The drawing under review shows one solid part. Ordinate dimensions are in mm from its lowest x, y, z. A direction names the side the tool comes from. Give positions to 0.01 mm unless a question says otherwise; leave off trailing zeros. Loops run counter-clockwise (first coordinate to the right, second up) from the corner with the lowest first, then second, coordinate; pieces in that order, holes last. Notation, with made-up numbers: M -38.5,44 L -16.5,44 A21 cw -16.5,78 Z; hole C -1,-9 d11. An arc over 180 degrees is marked long. Put each result on its own line as item: value. Start each with the question number.
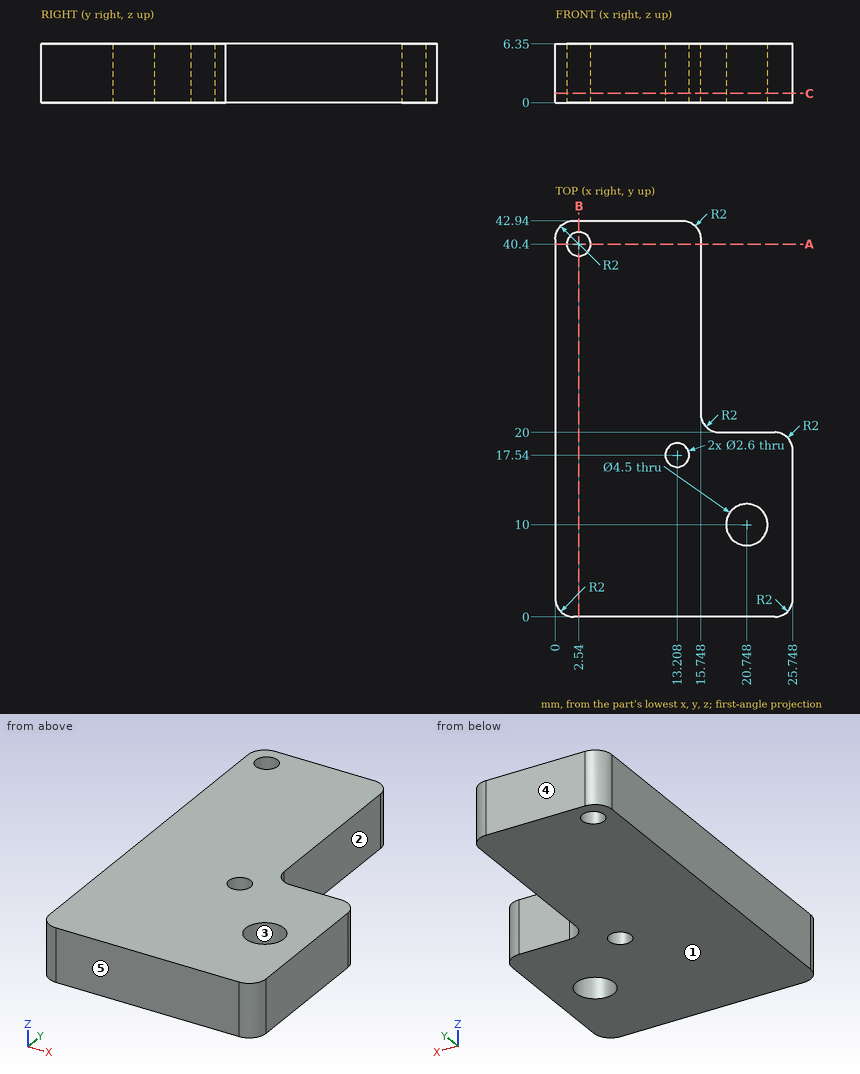
(1) Draft analysis for pull direction Y (two halves, no side actions). For the marked faces 3, 4 and 5, state which applies: +Y half, -Y half, draft (parallel to the pull), parting line (faces both ways), or undercut.
(2) To check wall thickness, follow L1, parallel to Y at x = 20.75, z = 5.75; L2, parallel to Y at x = 2.54, z = 2.5; L3, parallel to X at y = 25.5, z = 2.75. State the ranges of each line that lie inside material, in increasing order. Write a range as [from, to].
(3) We need section B-B, the plane x = 2.54. Write out the cut boundary in (y, z).
(4) We need section C-C, the plane z = 1. Write out the cut boundary in (x, y), plus the area to 3 significant figures.
(5) We need section A-A, the plane y = 40.4. Write out the cut boundary in (x, z), plus the area to 3 significant figures.
(6) For the marked faces 1 and 2, list the 3-axis set-ups (+Z, -Z, +X, -X, +Y, -Y) from which the entire face can be reached by the end or side of a thin tool; tool diameter is ignored.
(7) Insertion check: pin 1 (3.5 mm diameter, centred on x = 13.208, y = 17.54, fed in from +Z); pin 2 (1.6 mm diameter, centred on x = 2.54, y = 40.4, fed in from -Z); pin 3 (3 mm diameter, centred on y = 27.5, z = 2.5, fed in from +X). Each pin has a flat end and moves straight along its axis. Give the tip position at first contact, or say it passes through.
Check sheet entries:
1. face 3: undercut
1. face 4: +Y half
1. face 5: -Y half
2. L1: y = [0, 7.75], [12.25, 20]
2. L2: y = [0, 39.1], [41.7, 42.94]
2. L3: x = [0, 15.75]
3. outline: M 0,0 L 39.1,0 L 39.1,6.35 L 0,6.35 Z; M 41.7,0 L 42.94,0 L 42.94,6.35 L 41.7,6.35 Z
4. outline: M 0,2 A2 ccw 2,0 L 23.75,0 A2 ccw 25.75,2 L 25.75,18 A2 ccw 23.75,20 L 17.75,20 A2 cw 15.75,22 L 15.75,40.94 A2 ccw 13.75,42.94 L 2,42.94 A2 ccw 0,40.94 Z; hole C 2.54,40.4 d2.6; hole C 13.21,17.54 d2.6; hole C 20.75,10 d4.5
4. area: 846 mm²
5. outline: M 0,0 L 1.24,0 L 1.24,6.35 L 0,6.35 Z; M 3.84,0 L 15.75,0 L 15.75,6.35 L 3.84,6.35 Z
5. area: 83.5 mm²
6. face 1: -Z, +X, -X, +Y, -Y
6. face 2: +Z, -Z, +X, +Y
7. pin 1: stops at z = 6.35
7. pin 2: passes through
7. pin 3: stops at x = 15.75
